Can you work these out from the drawing? Everything is in mm from the part's minimum corner. Round coordinates to 2 decimals unless told otherwise and drop trailing zeros. Loops run counter-clockwise (first coordinate to the right, second up) from the corner with the lowest first, then second, coordinate; pieces in that order, holes last. Notation, with made-up numbers: M 14,60.25 L 27,60.25 A25 cw 27,80.25 Z; hole C 73,77 d11. An arc over 180 degrees is marked long. Use a Markdown table: item, result.
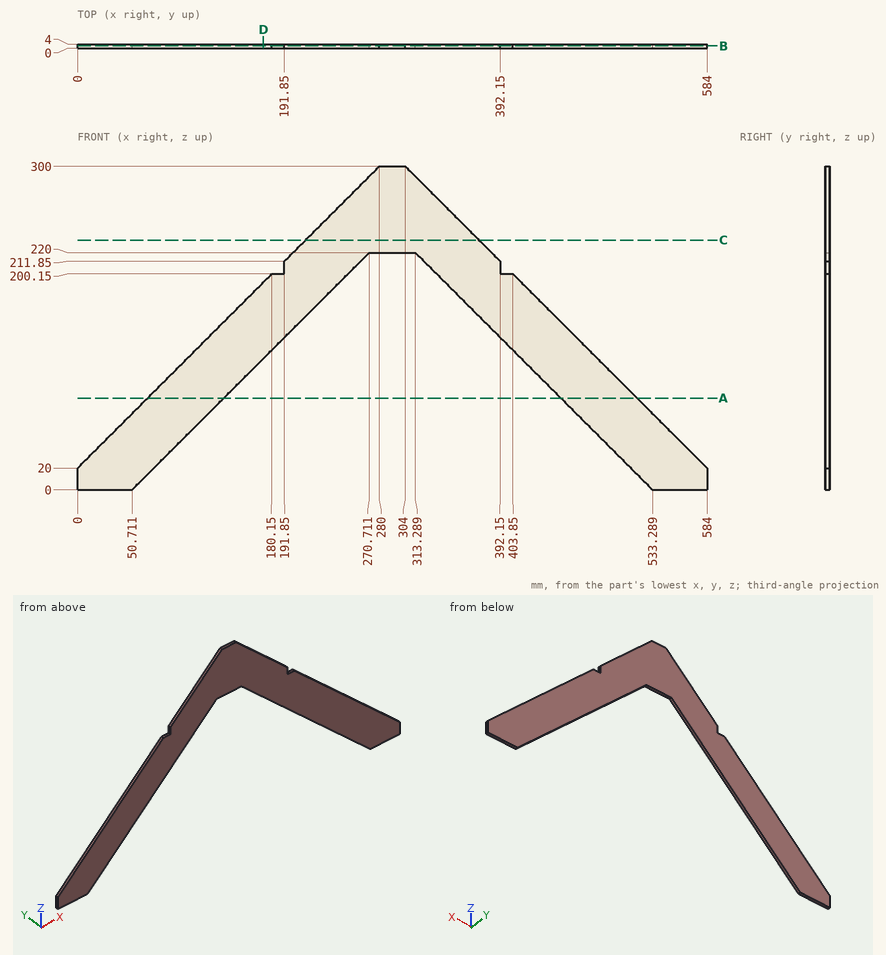
1. Imagine slicing it at B-B, the plane y = 2.15. Write out the boundary of the cut face in (x, z), then the cut area to 3 significant figures.
Answer sheet:
| item | result |
|---|---|
| outline | M 0,0 L 50.71,0 L 270.71,220 L 313.29,220 L 533.29,0 L 584,0 L 584,20 L 403.85,200.15 L 392.15,200.15 L 392.15,211.85 L 304,300 L 280,300 L 191.85,211.85 L 191.85,200.15 L 180.15,200.15 L 0,20 Z |
| area | 38,900 mm2 |
2. For pin 1 Ø1.2 at (y, z) = (2.5, 204) entering from -X; pin 2 Ø1.5 at (y, z) = (1.5, 155.5) entering from -X; pin 3 Ø8 at (x, z) = (151, 127.5) entering from -Y; pin 4 Ø2 at (y, z) = (1.5, 205.5) entering from +X, each with a flat end and sliding along its axis, tell me the tip position at first contact or that it passes through.
Answer sheet:
| item | result |
|---|---|
| pin 1 | x = 191.85 |
| pin 2 | x = 134.75 |
| pin 3 | y = 0 |
| pin 4 | x = 392.15 |
3. I need wall thicknesses on probe 1 along X at (y, z) = (2.4, 136.5); probe 2 along X at (y, z) = (3.25, 191); probe 3 along Z at (x, y) = (515, 0.7). Which ranges of each line are inside material? Lowest first, please. Write a range as from..to.
Answer sheet:
| item | result |
|---|---|
| probe 1 | 116.5..187.21, 396.79..467.5 |
| probe 2 | 171..241.71, 342.29..413 |
| probe 3 | 18.29..89 |
4. Imagine slicing it at D-D, the plane x = 172.5. Write out the boundary of the cut face in (y, z).
Answer sheet:
| item | result |
|---|---|
| outline | M 0,121.79 L 4,121.79 L 4,192.5 L 0,192.5 Z |
5. Imagine slicing it at A-A, the plane z = 85. Write out the boundary of the cut face in (x, y).
Answer sheet:
| item | result |
|---|---|
| outline | M 65,0 L 135.71,0 L 135.71,4 L 65,4 Z; M 448.29,0 L 519,0 L 519,4 L 448.29,4 Z |
6. Imagine slicing it at C-C, the plane z = 231.5. Write out the boundary of the cut face in (x, y), then the cut area to 3 significant figures.
Answer sheet:
| item | result |
|---|---|
| outline | M 211.5,0 L 372.5,0 L 372.5,4 L 211.5,4 Z |
| area | 644 mm2 |
